Check sheet for the modelled part. Datum: model origin and axes. Units: mm. Face numbers are marked on the shaded views. A direction names the side the tool comes from. Round coordinates to 2 decimals unless told otherwise and drop trailing zeros. Order: outer loops, then holes, each group sorted by start corner. A loop starts at its lowest first (then second) coordinate and runs counter-clockwise, first axis right, second up.
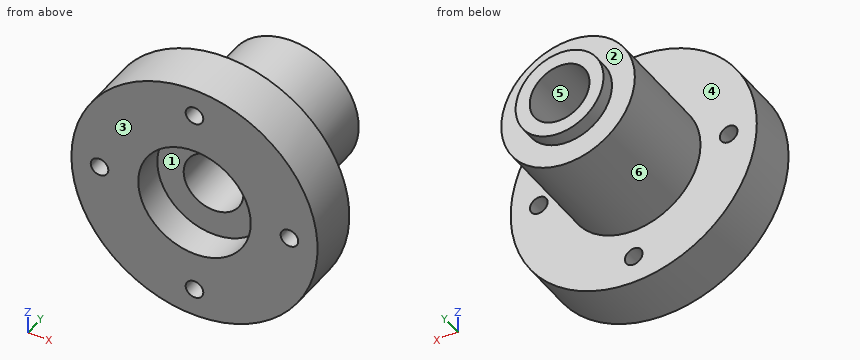
```python
from build123d import *

# Parameters (mm, degrees)
M6_TAPPED_HOLE1_D  = 5
SKETCH4_R          = 16
CUT_EXTRUDE1_DEPTH = 9


with BuildPart() as part:
    # Sketch1 → Revolve1 (revolve)
    with BuildSketch(Plane.XY):
        Polygon((-8.5, 0), (-35, 0), (-35, 15), (-19, 15), (-19, 46), (-12.5, 46), (-12.5, 50), (-8.5, 50), align=None)
    revolve(axis=Axis((0, 0, 0), (0, -1, 0)))

    # M6 Tapped Hole1 (through all)
    with Locations(Plane(origin=(0, 15, 0), x_dir=(1, 0, 0), z_dir=(0, 1, 0))):
        with Locations((-27, 0), (0, 27), (27, 0), (0, -27)):
            Hole(M6_TAPPED_HOLE1_D / 2)

    # Sketch4 → Cut-Extrude1 (cut)
    with BuildSketch(Plane.XZ):
        Circle(SKETCH4_R)
    extrude(amount=-CUT_EXTRUDE1_DEPTH, mode=Mode.SUBTRACT)


solid = part.part
```
Item 1: Release check for a two-part mould opening along X. For the marked faces 4, 5 and 6 record: released by +X, released by -X, zero draft, split by the parting line, or undercut.
Answer:
face 4: zero draft
face 5: undercut
face 6: split by the parting line
Item 2: Sectioned sample at C-C (x = 27). Record the cut outline in (y, z).
Answer:
outline: (0, -22.27) - (15, -22.27) - (15, -2.5) - (0, -2.5) - close; (0, 2.5) - (15, 2.5) - (15, 22.27) - (0, 22.27) - close
Item 3: Sectioned sample at B-B (z = 27). Record the cut outline in (x, y), and give its area (3 significant figures).
Answer:
outline: (-22.27, 0) - (-2.5, 0) - (-2.5, 15) - (-22.27, 15) - close; (2.5, 0) - (22.27, 0) - (22.27, 15) - (2.5, 15) - close
area: 593 mm2
Item 4: Sectioned sample at A-A (x = 0). Record the cut outline in (y, z), and give its area (3 significant figures).
Answer:
outline: (0, -35) - (15, -35) - (15, -29.5) - (0, -29.5) - close; (0, -24.5) - (15, -24.5) - (15, -19) - (46, -19) - (46, -12.5) - (50, -12.5) - (50, -8.5) - (9, -8.5) - (9, -16) - (0, -16) - close; (0, 16) - (9, 16) - (9, 8.5) - (50, 8.5) - (50, 12.5) - (46, 12.5) - (46, 19) - (15, 19) - (15, 24.5) - (0, 24.5) - close; (0, 29.5) - (15, 29.5) - (15, 35) - (0, 35) - close
area: 1,190 mm2
Item 5: Scan lines: line 1 along Z through (x, y) = (0, 10.75); line 2 along Y through (x, z) = (3.5, -20); line 3 along Y through (x, z) = (15, 8.5). Record each from-to range of solid material in increasing order.
Answer:
line 1: z = -35 to -29.5, -24.5 to -8.5, 8.5 to 24.5, 29.5 to 35
line 2: y = 0 to 15
line 3: y = 0 to 46
Item 6: Go/stop test with flat-tipped pins: P1, Ø4.5, axis at x = 27, z = 0, coming from the -Y side; P2, Ø6, axis at x = 0.5, z = 25.5, coming from the +Y side; P3, Ø1, axis at y = 9.5, z = 4.5, coming from the -X side; P4, Ø6, axis at x = 25.5, y = 7.5, coming from the -Z side. Record where each tip stops, or that it passes through.
Answer:
P1: passes through
P2: stops at y = 15
P3: stops at x = -34.77
P4: stops at z = -26.81
Item 7: Access from +Z, -Z, +X, -X, +Y, -Y to the whole of each face (thin tool, end or side, straight path). Record for the marked faces 1, 2 and 3.
Answer:
face 1: -Y
face 2: +Y
face 3: +Z, -Z, +X, -X, -Y
Item 8: Sectioned sample at D-D (y = 16). Record the cut outline in (x, z).
Answer:
outline: circle Ø38 at (0, 0); hole circle Ø17 at (0, 0)
